```python
from build123d import *

# Parameters (mm, degrees)
SKETCH_1_R          = 1.5
EXTRUDE_1_DEPTH     = 2
CUT_EXTRUDE_1_DEPTH = 2


with BuildPart() as part:
    # 草图1 → 凸台-拉伸1 (new body)
    with BuildSketch(Plane.XY):
        with BuildLine():
            Line((4, 0), (4, -75))
            Line((4, -75), (-4, -37.5))
            Line((-4, -37.5), (-4, 0))
            ThreePointArc((-4, 0), (0, 4), (4, 0))
        make_face()
        Circle(SKETCH_1_R, mode=Mode.SUBTRACT)
        with Locations((0, -10.66)):
            Circle(SKETCH_1_R, mode=Mode.SUBTRACT)
    extrude(amount=EXTRUDE_1_DEPTH)

    # 草图2 → 切除-拉伸1 (cut)
    with BuildSketch(Plane.XY.offset(2)):
        Polygon((4, -73.818025818), (3.747845508, -73.818025818), (4, -75), align=None)
    extrude(amount=-CUT_EXTRUDE_1_DEPTH, mode=Mode.SUBTRACT)


solid = part.part
```
CAD build for the part. Positions are in the model's coordinates, mm. Coordinates: 2 decimals unless noted, no trailing zeros. Write each loop counter-clockwise with the first axis right and the second up, starting at its lowest first coordinate (ties: lowest second). Pieces come first, ordered by that corner, then holes.
(1) Two-plate mould, pull along Y, no slides. Class faces 1 (the face through (-0.072, -55.913, 0.986)), 2 (the face through (-1.5, 0.07, 0.99)), 3 (the face through (0, 4, 1)), 4 (the face through (4, -36, 1)): +Y half, -Y half, draft (parallel to the pull), parting line (faces both ways), or undercut.
(2) Cut at B-B, the plane y = -10.66. List the corners of the cut face in (x, z), and give its area (3 significant figures).
(3) Cut at A-A, the plane z = 0.3. List the corners of the cut face in (x, y), and give its area (3 significant figures).
(4) Cut at D-D, the plane y = -64. List the corners of the cut face in (x, z), and give its area (3 significant figures).
(5) Cut at C-C, the plane x = 0.5. List the corners of the cut face in (y, z), and give its area (3 significant figures).
Geometry says:
1. face 1: -Y half
1. face 2: undercut
1. face 3: +Y half
1. face 4: draft
2. outline: (-4, 0) - (-1.5, 0) - (-1.5, 2) - (-4, 2) - close; (1.5, 0) - (4, 0) - (4, 2) - (1.5, 2) - close
2. area: 10.0 mm2
3. outline: (-4, -37.5) - (3.75, -73.82) - (4, -73.82) - (4, 0) arc R4 ccw to (-4, 0) - close; hole circle Ø3 at (0, -10.66); hole circle Ø3 at (0, 0)
3. area: 461 mm2
4. outline: (1.65, 0) - (4, 0) - (4, 2) - (1.65, 2) - close
4. area: 4.69 mm2
5. outline: (-58.59, 0) - (-12.07, 0) - (-12.07, 2) - (-58.59, 2) - close; (-9.25, 0) - (-1.41, 0) - (-1.41, 2) - (-9.25, 2) - close; (1.41, 0) - (3.97, 0) - (3.97, 2) - (1.41, 2) - close
5. area: 114 mm2
